Here's how the part is built. I have some questions about the finished solid (model axes, mm). A direction names the side the tool comes from. Round coordinates to 2 decimals unless told otherwise and drop trailing zeros. Write each loop counter-clockwise with the first axis right and the second up, starting at its lowest first coordinate (ties: lowest second). Pieces come first, ordered by that corner, then holes. Notation, with made-up numbers: (75.25, 32.25) -> (125.25, 32.25) arc R28 ccw to (125.25, 69.25) -> close; hole circle Ø3 at (6.25, 12.5). An arc over 180 degrees is marked (long way). Answer as CSV lines item,"result".
from build123d import *

# Parameters (mm, degrees)
F1_DEPTH     = 4
F2_DEPTH     = 15
F3_R         = 7
F4_SIZE      = 2
F5_W         = 19
F5_H         = 10
F5_W_2       = 4
F6_DEPTH     = 4
F7_T1_DEPTH  = 10
F7_T3_DEPTH  = 23.6580652273
F7_T5_DEPTH  = 23.6580652273
F7_T10_ANGLE = 16.8749432134
F7_T15_ANGLE = 13.853661309
F8_SIZE      = 3
F9_R         = 5


# Not quite as in the source:
# - a fillet or chamfer that OpenCascade refuses, or shapes differently, is made with other operations: its cross-section is extruded or revolved along the edge and cut away or added


with BuildPart() as f1:
    # F0 (on Front) → F1 (new body)
    with BuildSketch(Plane.XZ):
        Polygon((0, 0), (0, 60), (10, 60), (10, 20), (14, 20), (14, 64), (10, 64), (0, 64), (-4, 64), (-4, 0), align=None)
        with BuildLine():
            Line((-19, 0), (-4, 0))
            Line((-4, 0), (-4, 64))
            ThreePointArc((-4, 64), (53.018275741, 131.9517349578), (129.8387908342, 87.5993898895))
            Line((129.8387908342, 87.5993898895), (143.934180146, 92.7296920394))
            ThreePointArc((143.934180146, 92.7296920394), (50.413553076, 146.723851253), (-19, 64))
            Line((-19, 64), (-19, 0))
        make_face()
        with BuildLine():
            ThreePointArc((129.8387908342, 87.5993898895), (53.018275741, 131.9517349578), (-4, 64))
            Line((-4, 64), (0, 64))
            ThreePointArc((0, 64), (12.7505980895, 102.6652298584), (46, 126.1610810717))
            ThreePointArc((46, 126.1610810717), (94.0048047106, 122.1697627956), (126.0800203511, 86.2313093162))
            Line((126.0800203511, 86.2313093162), (129.8387908342, 87.5993898895))
        make_face()
        with BuildLine():
            Line((-23, 0), (-19, 0))
            Line((-19, 0), (-19, 64))
            ThreePointArc((-19, 64), (50.413553076, 146.723851253), (143.934180146, 92.7296920394))
            Line((143.934180146, 92.7296920394), (147.6929506292, 94.0977726127))
            ThreePointArc((147.6929506292, 94.0977726127), (49.7189603653, 150.6630822651), (-23, 64))
            Line((-23, 64), (-23, 0))
        make_face()
        Polygon((10, 64), (14, 64), (14, 92), (42, 92), (42, 52), (46, 52), (46, 92), (46, 96), (10, 96), (10, 92), align=None)
        with BuildLine():
            ThreePointArc((46, 126.1610810717), (12.7505980895, 102.6652298584), (0, 64))
            Line((0, 64), (10, 64))
            Line((10, 64), (10, 92))
            Line((10, 92), (10, 96))
            Line((10, 96), (46, 96))
            Line((46, 96), (46, 126.1610810717))
        make_face()
        Polygon((137.9303256941, 65.3680805733), (129.8387908342, 87.5993898895), (126.0800203511, 86.2313093162), (134.1715552109, 64), align=None)
        Polygon((143.934180146, 92.7296920394), (129.8387908342, 87.5993898895), (137.9303256941, 65.3680805733), (152.0257150059, 70.4983827232), align=None)
        Polygon((147.6929506292, 94.0977726127), (143.934180146, 92.7296920394), (152.0257150059, 70.4983827232), (155.784485489, 71.8664632965), align=None)
    extrude(amount=-F1_DEPTH)

    # F0 (on Front) → F2 (join)
    with BuildSketch(Plane.XZ):
        Polygon((0, 0), (0, 60), (10, 60), (10, 20), (14, 20), (14, 64), (10, 64), (0, 64), (-4, 64), (-4, 0), align=None)
        with BuildLine():
            ThreePointArc((129.8387908342, 87.5993898895), (53.018275741, 131.9517349578), (-4, 64))
            Line((-4, 64), (0, 64))
            ThreePointArc((0, 64), (12.7505980895, 102.6652298584), (46, 126.1610810717))
            ThreePointArc((46, 126.1610810717), (94.0048047106, 122.1697627956), (126.0800203511, 86.2313093162))
            Line((126.0800203511, 86.2313093162), (129.8387908342, 87.5993898895))
        make_face()
        with BuildLine():
            Line((-23, 0), (-19, 0))
            Line((-19, 0), (-19, 64))
            ThreePointArc((-19, 64), (50.413553076, 146.723851253), (143.934180146, 92.7296920394))
            Line((143.934180146, 92.7296920394), (147.6929506292, 94.0977726127))
            ThreePointArc((147.6929506292, 94.0977726127), (49.7189603653, 150.6630822651), (-23, 64))
            Line((-23, 64), (-23, 0))
        make_face()
        Polygon((147.6929506292, 94.0977726127), (143.934180146, 92.7296920394), (152.0257150059, 70.4983827232), (155.784485489, 71.8664632965), align=None)
        Polygon((137.9303256941, 65.3680805733), (129.8387908342, 87.5993898895), (126.0800203511, 86.2313093162), (134.1715552109, 64), align=None)
        Polygon((10, 64), (14, 64), (14, 92), (42, 92), (42, 52), (46, 52), (46, 92), (46, 96), (10, 96), (10, 92), align=None)
    extrude(amount=F2_DEPTH)

    # F3
    f3_edges = [f1.edges().sort_by_distance(p)[0] for p in [
        (50.413553, 0, 146.723851),
        (53.018276, 0, 131.951735),
        (133.884558, 0, 76.483735),
        (147.979948, 0, 81.614037),
        (-19, 0, 32),
        (-4, 0, 32),
    ]]
    fillet(f3_edges, radius=F3_R)

    # F4
    f4_edges = [f1.edges().sort_by_distance(p)[0] for p in [
        (130.125788, 4, 75.115655),
        (151.738718, 4, 82.982118),
        (0, 4, 30),
        (94.004805, 4, 122.169763),
        (49.71896, 4, 150.663082),
        (-23, 4, 32),
    ]]
    chamfer(f4_edges, length=F4_SIZE)

    # F5 (on face) → F6 (join)
    with BuildSketch(Plane.XZ.offset(15)):
        Polygon((137.9303256941, 65.3680805733), (129.8387908342, 87.5993898895), (126.0800203511, 86.2313093162), (134.1715552109, 64), align=None)
        Polygon((147.6929506292, 94.0977726127), (129.8387908342, 87.5993898895), (137.9303256941, 65.3680805733), (155.784485489, 71.8664632965), align=None)
        with Locations((-13.5, 5)):
            Rectangle(F5_W, F5_H)
        with Locations((-2, 5)):
            Rectangle(F5_W_2, F5_H)
        with BuildLine():
            Line((143.7370980696, 103.2997377546), (125.7340390711, 96.7471601534))
            ThreePointArc((125.7340390711, 96.7471601534), (127.95279444, 92.2479321755), (129.8387908342, 87.5993898895))
            Line((129.8387908342, 87.5993898895), (147.6929506292, 94.0977726127))
            ThreePointArc((147.6929506292, 94.0977726127), (145.8460524475, 98.7550831341), (143.7370980696, 103.2997377546))
        make_face()
        with BuildLine():
            ThreePointArc((129.8387908342, 87.5993898895), (127.95279444, 92.2479321755), (125.7340390711, 96.7471601534))
            Line((125.7340390711, 96.7471601534), (121.932649899, 95.3635676459))
            ThreePointArc((121.932649899, 95.3635676459), (124.1827434345, 90.8775534519), (126.0800203511, 86.2313093162))
            Line((126.0800203511, 86.2313093162), (129.8387908342, 87.5993898895))
        make_face()
    extrude(amount=F6_DEPTH)

    # F7: chamfer of 4 on 6 edges, made by hand

    # F7_s2 → F7_t1 (join)
    with BuildSketch(Plane.XY):
        Polygon((-15, -15), (-19, -11), (-19, -15), align=None)
        Polygon((-8, -15), (-4, -11), (-4, -15), align=None)
    extrude(amount=F7_T1_DEPTH)

    # F7_s4 → F7_t3 (join)
    with BuildSketch(Plane(origin=(-12.9656479113, 0, 35.622824865), x_dir=(0, 1, 0), z_dir=(0.3420201433, 0, -0.9396926208))):
        Polygon((-11, 166.9693095239), (-15, 162.9693095239), (-15, 166.9693095239), align=None)
    extrude(amount=F7_T3_DEPTH)

    # F7_s6 → F7_t5 (join)
    with BuildSketch(Plane(origin=(-4.8741130515, 0, 13.3915155488), x_dir=(0, 1, 0), z_dir=(-0.3420201433, 0, 0.9396926208))):
        Polygon((-11, -151.9693095239), (-15, -155.9693095239), (-15, -151.9693095239), align=None)
    extrude(amount=F7_T5_DEPTH)


with BuildPart() as f7_tool8:
    # F7_s9 → F7_t10 (revolve)
    with BuildSketch(Plane(origin=(-12.9656479113, 0, 35.622824865), x_dir=(0, 1, 0), z_dir=(0.3420201433, 0, -0.9396926208))):
        Polygon((-11, 151.9693095239), (-15, 155.9693095239), (-15, 151.9693095239), align=None)
    revolve(axis=Axis((65, -15, 64), (0, -1, 0)), revolution_arc=F7_T10_ANGLE)

    split(bisect_by=Plane(origin=(-16.3858493446, 0, 45.0197510729), x_dir=(0, 1, 0), z_dir=(0.3420201433, 0, -0.9396926208)), keep=Keep.TOP)


with BuildPart() as f1_1:
    add(f1.part)

    # F7_t7: union F7_tool8
    add(f7_tool8.part)


with BuildPart() as f7_tool13:
    # F7_s14 → F7_t15 (revolve)
    with BuildSketch(Plane(origin=(-9.4367447279, 0, 14.0679214359), x_dir=(0, 1, 0), z_dir=(-0.5570736436, 0, 0.830463097))):
        Polygon((-11, -173.6328145012), (-15, -169.6328145012), (-15, -173.6328145012), align=None)
    revolve(axis=Axis((65, -15, 64), (0, 1, 0)), revolution_arc=F7_T15_ANGLE)

    split(bisect_by=Plane(origin=(-16.3858493446, 0, 45.0197510729), x_dir=(0, 1, 0), z_dir=(0.3420201433, 0, -0.9396926208)), keep=Keep.TOP)


with BuildPart() as f1_2:
    add(f1_1.part)

    # F7_t12: union F7_tool13
    add(f7_tool13.part)

    # F8
    f8_edges = [f1_2.edges().sort_by_distance(p)[0] for p in [
        (-23, -19, 5),
        (0, -19, 5),
        (124.182743, -19, 90.877553),
        (145.846052, -19, 98.755083),
        (130.125788, -19, 75.115655),
        (151.738718, -19, 82.982118),
    ]]
    chamfer(f8_edges, length=F8_SIZE)

    # F9
    f9_edges = [f1_2.edges().sort_by_distance(p)[0] for p in [
        (42, -5.5, 92),
        (14, -5.5, 92),
    ]]
    fillet(f9_edges, radius=F9_R)


solid = f1_2.part
Item 1: Suppose I cut it at A-A, the plane z = 42. List the corners of the cut face in (x, y) for me, then the cut area to 3 significant figures.
Results found:
outline,"(-23, -15) -> (-19, -15) -> (-19, -7) arc R7 cw to (-12, 0) -> (-11, 0) arc R7 cw to (-4, -7) -> (-4, -15) -> (0, -15) -> (0, 2) -> (-2, 4) -> (-21, 4) -> (-23, 2) -> close; (10, -15) -> (14, -15) -> (14, 4) -> (10, 4) -> close"
area,"305 mm²"
Item 2: I need wall thicknesses on L1, parallel to X at y = -1.25, z = 55; L2, parallel to X at y = -9.75, z = 13.5; L3, parallel to X at y = -4.5, z = 106. Which ranges of each line are inside material? Lowest first, please.
Results found:
L1,"x = -23 to -15.99, -7.01 to 0, 10 to 14, 42 to 46"
L2,"x = -23 to -19, -4 to 0"
L3,"x = -12.33 to -7.21, 9.67 to 15.39, 114.61 to 120.33, 137.21 to 142.33"
Item 3: If we mould it in two halves opening along Y, with no side actions, what happens to faces 1 (the cylindrical face through (146.06, -2, 80.74)), 2 (the flat face through (150.843, 3.014, 82.48)), 3 (the flat face through (130.07, -6.87, 75.27))? For each: pulls with the +Y half, pulls with the -Y half, needs draft (parallel to the pull), parting line crosses it, or undercut.
Results found:
face 1,"undercut"
face 2,"pulls with the +Y half"
face 3,"needs draft"
Item 4: Will these pins go through, and if not, where does the flat tip stop? pin 1 (3 mm diameter, centred on x = 35, y = -6, fed in from -Z); pin 2 (2 mm diameter, centred on x = 12, y = -10, fed in from -Z); pin 3 (9.5 mm diameter, centred on y = -8, z = 39.5, fed in from +X).
Results found:
pin 1,"stops at z = 92"
pin 2,"stops at z = 20"
pin 3,"stops at x = 14"
Item 5: For faces 4 (the conical face through (140.09, -13.03, 96.87)), 5 (the flat face through (147.923, -8.972, 81.77)), 6 (the conical face through (144.41, -17.52, 98.25)), 7 (the flat face through (44, -5, 52)), 8 (the flat face through (10, -5, 40)), which set-ups out of +Z, -Z, +X, -X, +Y, -Y let a thin tool reach every point of the face, with its end or its side?
Results found:
face 4,"none"
face 5,"-Z"
face 6,"+Z, +X, -Y"
face 7,"-Z, +X, +Y, -Y"
face 8,"-Z, +Y, -Y"
